```python
from build123d import *

# Parameters (mm, degrees)
F0_W     = 60
F0_H     = 30
F1_DEPTH = 35
F2_DEPTH = 30
F4_W     = 60
F4_H     = 30
F4_R     = 12.5
F5_DEPTH = 30
F7_D     = 3.4
F8_D     = 5.5


with BuildPart() as f1:
    # F0 (on Top) → F1 (new body)
    with BuildSketch(Plane.XY):
        Rectangle(F0_W, F0_H)
        with BuildLine():
            ThreePointArc((-2.5, -6.5383484153), (-3.9686269666, 5.7662812973), (7, 0))
            ThreePointArc((7, 0), (5.7662812973, -3.9686269666), (2.5, -6.5383484153))
            Line((2.5, -6.5383484153), (2.5, -9.5))
            Line((2.5, -9.5), (0, -9.5))
            Line((0, -9.5), (-2.5, -9.5))
            Line((-2.5, -9.5), (-2.5, -6.5383484153))
        make_face(mode=Mode.SUBTRACT)
        with BuildLine():
            ThreePointArc((2.5, -6.5383484153), (5.7662812973, -3.9686269666), (7, 0))
            ThreePointArc((7, 0), (-3.9686269666, 5.7662812973), (-2.5, -6.5383484153))
            ThreePointArc((-2.5, -6.5383484153), (0, -7), (2.5, -6.5383484153))
        make_face()
        with BuildLine():
            ThreePointArc((2.5, -6.5383484153), (0, -7), (-2.5, -6.5383484153))
            Line((-2.5, -6.5383484153), (-2.5, -9.5))
            Line((-2.5, -9.5), (0, -9.5))
            Line((0, -9.5), (2.5, -9.5))
            Line((2.5, -9.5), (2.5, -6.5383484153))
        make_face()
    extrude(amount=F1_DEPTH)

    # F0 (on Top) → F2 (cut)
    with BuildSketch(Plane.XY):
        with BuildLine():
            ThreePointArc((2.5, -6.5383484153), (5.7662812973, -3.9686269666), (7, 0))
            ThreePointArc((7, 0), (-3.9686269666, 5.7662812973), (-2.5, -6.5383484153))
            ThreePointArc((-2.5, -6.5383484153), (0, -7), (2.5, -6.5383484153))
        make_face()
        with BuildLine():
            ThreePointArc((2.5, -6.5383484153), (0, -7), (-2.5, -6.5383484153))
            Line((-2.5, -6.5383484153), (-2.5, -9.5))
            Line((-2.5, -9.5), (0, -9.5))
            Line((0, -9.5), (2.5, -9.5))
            Line((2.5, -9.5), (2.5, -6.5383484153))
        make_face()
    extrude(amount=F2_DEPTH, mode=Mode.SUBTRACT)

    # F4 (on face) → F5 (cut)
    with BuildSketch(Plane.XY):
        Rectangle(F4_W, F4_H)
        Circle(F4_R, mode=Mode.SUBTRACT)
    extrude(amount=F5_DEPTH, mode=Mode.SUBTRACT)

    # F7 (through all)
    with Locations(Plane.XY.offset(35)):
        with Locations((-18.5, 0), (18.5, 0)):
            Hole(F7_D / 2)

    # F8 (through all)
    with Locations(Plane(origin=(0, 0, 0), x_dir=(1, 0, 0), z_dir=(0, 0, -1))):
        with Locations((0, 0)):
            Hole(F8_D / 2)


solid = f1.part
```
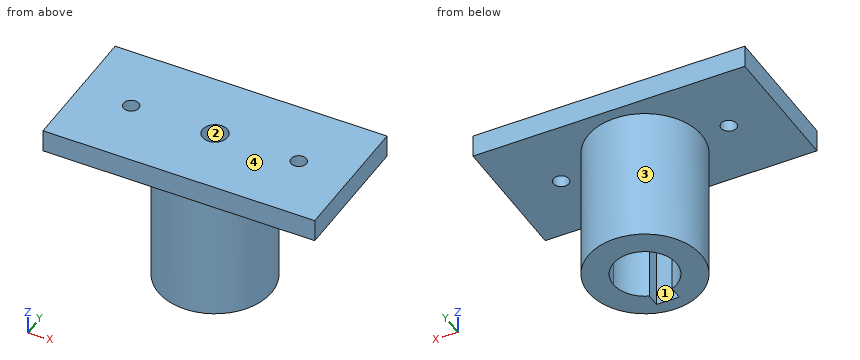
Source: CAD feature listing. Evaluate the final solid. Frame: model axes, mm. Face numbers are marked on the shaded views. Give positions to 0.01 mm unless a question says otherwise; leave off trailing zeros. Loops run counter-clockwise (first coordinate to the right, second up) from the corner with the lowest first, then second, coordinate; pieces in that order, holes last. Notation, with made-up numbers: (26.25, 73) -> (39.25, 73) arc R15 ccw to (39.25, 97) -> close; hole circle Ø10 at (81.5, 63). An arc over 180 degrees is marked (long way). Put each result on its own line as item: value. Start each with the question number.
1) Cut plane D-D (y = 4.75). Return loops of the section in (x, z).
2) Cut plane A-A (x = 0). Return loops of the section in (y, z), then the cut area to 4 significant figures.
3) Material intervals for probe 1 along Y at (x, z) = (0, 12); probe 2 along Y at (x, z) = (-18.5, 33.3); probe 3 along Z at (x, y) = (-0.5, 4), sorted ascending.
4) Draft query along X for the marked faces 1, 2, 3 and 4. Return one class per face: released by +X, released by -X, zero draft, split by the parting line, or undercut.
5) Cut plane B-B (z = 31.5). Return loops of the section in (x, y), then the cut area to 3 significant figures.
6) Contact query for flat-ended pins moving along their axis: P1, Ø11, axis at x = 0, y = 0, coming from the -Z side; P2, Ø2, axis at y = 4, z = 10.5, coming from the -X side; P3, Ø12, axis at x = 16.5, z = 12, coming from the -Y side; P4, Ø3.5, axis at x = 0, y = 0, coming from the -Z side. Output: stop coordinate, or through.
7) Cut plane C-C (z = 25). Return loops of the section in (x, y).
Results are:
1. outline: (-30, 30) -> (-11.56, 30) -> (-11.56, 0) -> (-5.14, 0) -> (-5.14, 30) -> (5.14, 30) -> (5.14, 0) -> (11.56, 0) -> (11.56, 30) -> (30, 30) -> (30, 35) -> (-30, 35) -> close
2. outline: (-15, 30) -> (-12.5, 30) -> (-12.5, 0) -> (-9.5, 0) -> (-9.5, 30) -> (-2.75, 30) -> (-2.75, 35) -> (-15, 35) -> close; (2.75, 30) -> (7, 30) -> (7, 0) -> (12.5, 0) -> (12.5, 30) -> (15, 30) -> (15, 35) -> (2.75, 35) -> close
2. area: 377.5 mm2
3. probe 1: y = -12.5 to -9.5, 7 to 12.5
3. probe 2: y = -15 to -1.7, 1.7 to 15
3. probe 3: z = 30 to 35
4. face 1: undercut
4. face 2: undercut
4. face 3: split by the parting line
4. face 4: zero draft
5. outline: (-30, -15) -> (30, -15) -> (30, 15) -> (-30, 15) -> close; hole circle Ø3.4 at (-18.5, 0); hole circle Ø5.5 at (0, 0); hole circle Ø3.4 at (18.5, 0)
5. area: 1,760 mm2
6. P1: stops at z = 30
6. P2: stops at x = -12.13
6. P3: stops at y = -6.78
6. P4: passes through
7. outline: circle Ø25 at (0, 0); hole (-2.5, -9.5) -> (2.5, -9.5) -> (2.5, -6.54) arc R7 ccw (long way) to (-2.5, -6.54) -> close
